Source: three-view drawing plus pictorial views. Frame: mm from the lowest corner of the part. Coordinates: 2 decimals unless noted, no trailing zeros. Loops run counter-clockwise (first coordinate to the right, second up) from the corner with the lowest first, then second, coordinate; pieces in that order, holes last. Notation, with made-up numbers: (36.5, -2.5) - (72.5, -2.5) arc R24 ccw to (72.5, 19.5) - close; hole circle Ø5 at (-26.5, 77.5). An arc over 180 degrees is marked (long way). Return JSON: item names as keys, results as strings.
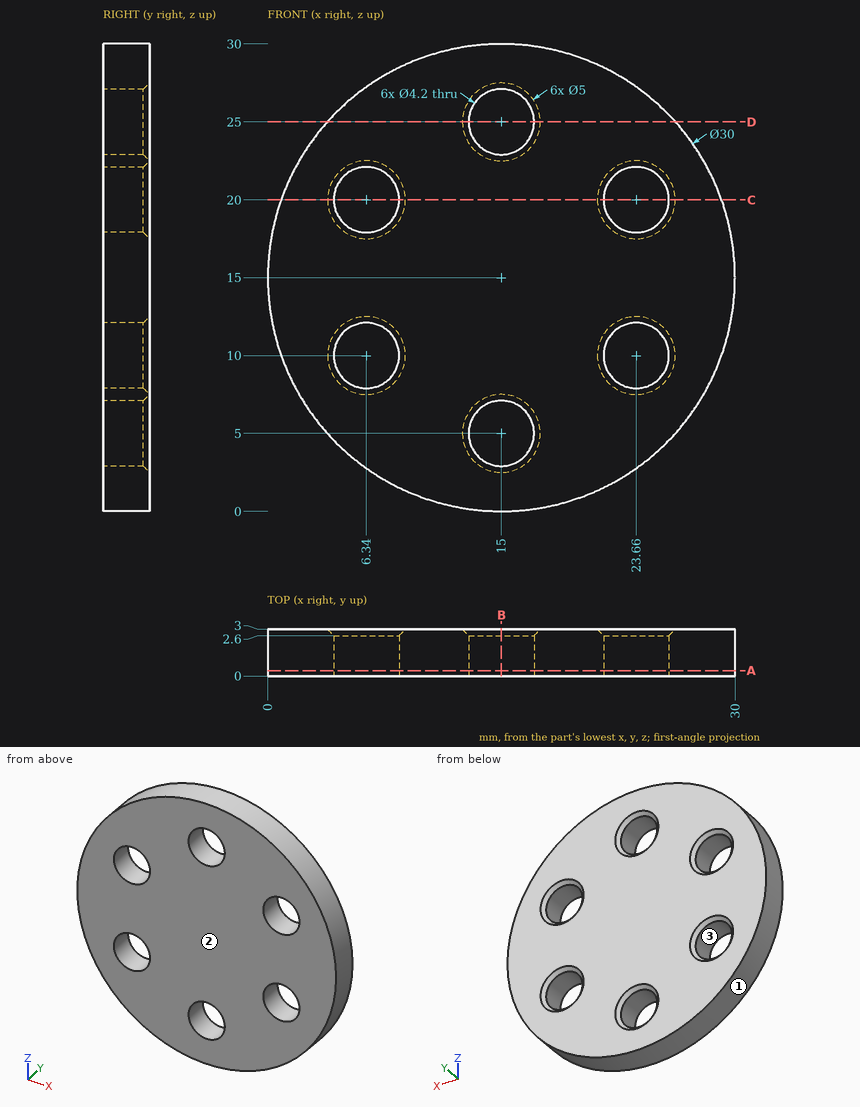
Item 1: Section query A-A, the plane y = 0.35. Return loops of the section in (x, z).
Worked out:
{"outline": "circle Ø30 at (15, 15); hole circle Ø4.2 at (6.34, 10); hole circle Ø4.2 at (6.34, 20); hole circle Ø4.2 at (15, 5); hole circle Ø4.2 at (15, 25); hole circle Ø4.2 at (23.66, 10); hole circle Ø4.2 at (23.66, 20)"}
Item 2: First-contact query: pin 1 Ø1.5 at (x, z) = (24.5, 10) entering from +Y; pin 2 Ø5.5 at (x, z) = (6.34, 10) entering from +Y; pin 3 Ø1.5 at (x, z) = (16, 4) entering from +Y (1 decimal); pin 4 Ø1 at (y, z) = (1.5, 7) entering from -X. Flat tips, straight axial feed; report the tip coordinate or a pass-through.
Worked out:
{"pin 1": "through", "pin 2": "y = 3", "pin 3": "y = 2.7", "pin 4": "x = 2.01"}
Item 3: Section query C-C, the plane z = 20. Return loops of the section in (x, y).
Worked out:
{"outline": "(0.86, 0) - (4.24, 0) - (4.24, 2.6) - (3.84, 3) - (0.86, 3) - close; (8.44, 0) - (21.56, 0) - (21.56, 2.6) - (21.16, 3) - (8.84, 3) - (8.44, 2.6) - close; (25.76, 0) - (29.14, 0) - (29.14, 3) - (26.16, 3) - (25.76, 2.6) - close"}
Item 4: Section query B-B, the plane x = 15. Return loops of the section in (y, z).
Worked out:
{"outline": "(0, 0) - (3, 0) - (3, 2.5) - (2.6, 2.9) - (0, 2.9) - close; (0, 7.1) - (2.6, 7.1) - (3, 7.5) - (3, 22.5) - (2.6, 22.9) - (0, 22.9) - close; (0, 27.1) - (2.6, 27.1) - (3, 27.5) - (3, 30) - (0, 30) - close"}
Item 5: Mould query, pull axis X, two halves, no side actions, for the marked faces 1, 2 and 3. Classes: +X half, -X half, draft (parallel to the pull), parting line (faces both ways), or undercut.
Worked out:
{"face 1": "parting line", "face 2": "draft", "face 3": "undercut"}
Item 6: Section query D-D, the plane z = 25. Return loops of the section in (x, y).
Worked out:
{"outline": "(3.82, 0) - (12.9, 0) - (12.9, 2.6) - (12.5, 3) - (3.82, 3) - close; (17.1, 0) - (26.18, 0) - (26.18, 3) - (17.5, 3) - (17.1, 2.6) - close"}
Item 7: Ray query, probe 1 along Z at (x, y) = (15, 1.2); probe 2 along X at (y, z) = (2.3, 19.75) (1 decimal); probe 3 along X at (y, z) = (0.4, 21.75) (1 decimal). Return the intervals inside material, ascending. Write a range as from..to.
Worked out:
{"probe 1": "0..2.9, 7.1..22.9, 27.1..30", "probe 2": "0.8..4.3, 8.4..21.6, 25.7..29.2", "probe 3": "1.6..5.2, 7.5..22.5, 24.8..28.4"}
